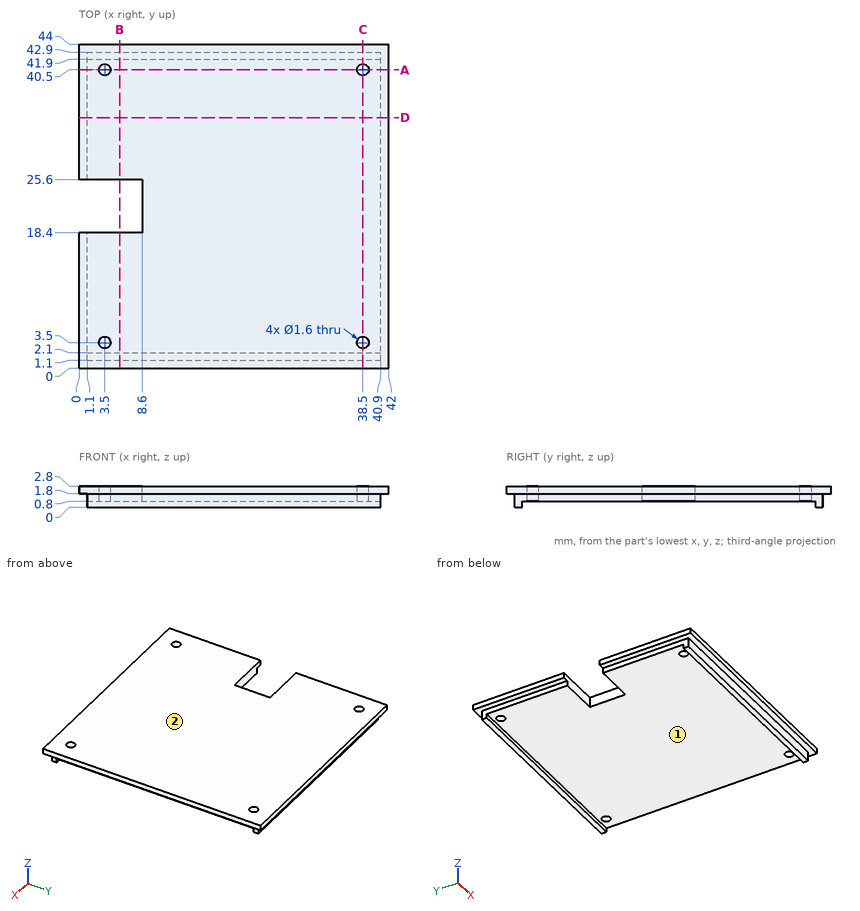
Check sheet for the drawn part. Datum: minimum x, y, z corner. Units: mm. Give positions to 0.01 mm unless a question says otherwise; leave off trailing zeros. Order: outer loops, then holes, each group sorted by start corner. A loop starts at its lowest first (then second) coordinate and runs counter-clockwise, first axis right, second up. Notation, with made-up numbers: (-24.75, 84.25) - (21.25, 84.25) arc R8 cw to (21.25, 95.25) - close; hole circle Ø2 at (-20, 83.25). An arc over 180 degrees is marked (long way). Write item = value, one per line. Start each with the question number.
1) Section check D-D (y = 34). Enter the section's corners in (x, z).
2) Gauge pin test, flat ends, axial feed: pin 1 Ø0.9 at (y, z) = (7.5, 1) entering from -X; pin 2 Ø1.4 at (y, z) = (13, 1) entering from +X; pin 3 Ø2 at (x, y) = (38.5, 3.5) entering from -Z. Record the tip position at first contact, or that the pin passes through.
3) Draft check along Y on the marked faces 1 and 2. Enter one of: released by +Y, released by -Y, zero draft, split by the parting line, or undercut.
4) Scan lines: L1, parallel to X at y = 3.5, z = 2.1; L2, parallel to X at y = 3.5, z = 1.3; L3, parallel to Y at x = 38.5, z = 2.05. Record each from-to range of solid material in increasing order.
5) Section check C-C (x = 38.5). Enter the section's corners in (y, z), then the cut area to 3 significant figures.
6) Section check A-A (y = 40.5). Enter the section's corners in (x, z), then the cut area to 3 significant figures.
7) Section check B-B (x = 5.5). Enter the section's corners in (y, z).
Geometry check:
q1.outline = (0, 1.8) - (1.1, 1.8) - (1.1, 0.8) - (40.9, 0.8) - (40.9, 1.8) - (42, 1.8) - (42, 2.8) - (0, 2.8) - close
q2.pin_1 = 1.1
q2.pin_2 = 40.9
q2.pin_3 = 0.8
q3.face_1 = undercut
q3.face_2 = zero draft
q4.L1 = 0 to 2.7, 4.3 to 37.7, 39.3 to 42
q4.L2 = 1.1 to 2.7, 4.3 to 37.7, 39.3 to 40.9
q4.L3 = 0 to 2.7, 4.3 to 39.7, 41.3 to 44
q5.outline = (0, 1.8) - (1.1, 1.8) - (1.1, 0) - (2.1, 0) - (2.1, 0.8) - (2.7, 0.8) - (2.7, 2.8) - (0, 2.8) - close; (4.3, 0.8) - (39.7, 0.8) - (39.7, 2.8) - (4.3, 2.8) - close; (41.3, 0.8) - (41.9, 0.8) - (41.9, 0) - (42.9, 0) - (42.9, 1.8) - (44, 1.8) - (44, 2.8) - (41.3, 2.8) - close
q5.area = 81.0 mm2
q6.outline = (0, 1.8) - (1.1, 1.8) - (1.1, 0.8) - (2.7, 0.8) - (2.7, 2.8) - (0, 2.8) - close; (4.3, 0.8) - (37.7, 0.8) - (37.7, 2.8) - (4.3, 2.8) - close; (39.3, 0.8) - (40.9, 0.8) - (40.9, 1.8) - (42, 1.8) - (42, 2.8) - (39.3, 2.8) - close
q6.area = 75.4 mm2
q7.outline = (0, 1.8) - (1.1, 1.8) - (1.1, 0) - (2.1, 0) - (2.1, 0.8) - (18.4, 0.8) - (18.4, 2.8) - (0, 2.8) - close; (25.6, 0.8) - (41.9, 0.8) - (41.9, 0) - (42.9, 0) - (42.9, 1.8) - (44, 1.8) - (44, 2.8) - (25.6, 2.8) - close
